The listing builds one solid part. Answer for the finished solid, in the listing's coordinates (mm). A direction names the side the tool comes from. Coordinates: 2 decimals unless noted, no trailing zeros. Order: outer loops, then holes, each group sorted by start corner. A loop starts at its lowest first (then second) coordinate and runs counter-clockwise, first axis right, second up. Notation, with made-up numbers: (70, 59.5) - (111, 59.5) arc R32 cw to (111, 96.5) - close; hole circle Ø2 at (67, 84.25). An arc over 180 degrees is marked (long way). Use a Markdown table: item, result. Add a question column.
Item 1: The part is cut by section B-B, the plane z = 5. Give the vertices of the cut face in (x, y), then the cut area to 3 significant figures.
Item 2: The part is cut by section A-A, the plane x = -33. Give the vertices of the cut face in (y, z), then the cut area to 3 significant figures.
Item 3: Find the intervals of material crossed by line 1 along X through (y, z) = (2.5, 3); line 2 along Y through (x, z) = (37.5, -2.5); line 3 along Y through (x, z) = (18.5, -9), in increasing order.
Item 4: Flat-ended cylindrical pins translate along their axes: P1, Ø3, axis at x = 15.5, z = 22, coming from the +Y side; P2, Ø10, axis at x = -1, y = 31.5, coming from the -Z side; P3, Ø12, axis at x = -4.5, y = 9.5, coming from the +Z side. Find the tip coordinate at first contact, or state that the pin passes through.
Item 5: For faces 1 (the flat face through (-1.29, 7.19, 0.91)), 2 (the flat face through (-10.32, -0.54, 6.53)), 3 (the cylindrical face through (32.9, 3.5, -23.5)), determine the directions among +Z, -Z, +X, -X, +Y, -Y from which every point of the face is accessible in a straight line to the end or side of a thin tool.
Item 6: The part is cut by section D-D, the plane z = 25. Give the vertices of the cut face in (x, y), then the cut area to 3 significant figures.
Item 7: The part is cut by section C-C, the plane y = 3.5. Give the vertices of the cut face in (x, z).
Item 8: The mould has two halves that part along Y. Classify faces 4 (the flat face through (7.42, 17.14, -4.5)), 5 (the flat face through (39, 3, 26)), 6 (the flat face through (-4.37, 22.4, 1.41)), 7 (the flat face through (9.5, 29.32, -7.2)): released by +Y, released by -Y, zero draft, split by the parting line, or undercut.
from build123d import *

# Parameters (mm, degrees)
BOSS_EXTRUDE1_DEPTH = 7
EXTRUDE_THIN1_DEPTH = 7
SKETCH4_R           = 4
BOSS_EXTRUDE2_DEPTH = 4


with BuildPart() as part:
    # Sketch1 → Boss-Extrude1 (new body)
    with BuildSketch(Plane(origin=(0, 0, 0), x_dir=(1, 0, 0), z_dir=(0, 1, 0))):
        Polygon((34, 31), (44, 21), (44, -21), (34, -31), (-34, -31), (-44, -21), (-44, 21), (-34, 31), align=None)
        with BuildLine():
            Line((-30, 20.5), (-30, -20.5))
            ThreePointArc((-30, -20.5), (-33, -23.5), (-36, -20.5))
            Line((-36, -20.5), (-36, 20.5))
            ThreePointArc((-36, 20.5), (-33, 23.5), (-30, 20.5))
        make_face(mode=Mode.SUBTRACT)
        with BuildLine():
            Line((36, 20.5), (36, -20.5))
            ThreePointArc((36, -20.5), (33, -23.5), (30, -20.5))
            Line((30, -20.5), (30, 20.5))
            ThreePointArc((30, 20.5), (33, 23.5), (36, 20.5))
        make_face(mode=Mode.SUBTRACT)
    extrude(amount=BOSS_EXTRUDE1_DEPTH)

    # Sketch3 → Extrude-Thin1 (add, symmetric)
    with BuildSketch(Plane(origin=(0, 0, 0), x_dir=(0.849441251, 0, -0.527683201), z_dir=(0.527683201, 0, 0.849441251))):
        Polygon((-18.849066913, 7), (8.678571497, 27), (8.678571497, 7), (-1.321428503, 7), (-1.321428503, 7.373894945), (-12.97121439, -1.090169944), align=None)
    extrude(amount=EXTRUDE_THIN1_DEPTH, both=True)

    # Sketch4 → Boss-Extrude2 (add)
    with BuildSketch(Plane(origin=(-8.359258135, 13.544823437, 5.192872478), x_dir=(0.866435488, 0.466201263, 0.178734239), z_dir=(-0.49928904, 0.809016994, 0.310164404))):
        with BuildLine():
            Line((20.238219538, 24.365708041), (-17.853578159, -4.883475366))
            Line((-17.853578159, -4.883475366), (-9.327190536, -15.987560835))
            Line((-9.327190536, -15.987560835), (28.764607161, 13.261622572))
            ThreePointArc((28.764607161, 13.261622572), (30.053456084, 23.076859118), (20.238219538, 24.365708041))
        make_face()
        with Locations((24.501413349, 18.813665306)):
            Circle(SKETCH4_R, mode=Mode.SUBTRACT)
    extrude(amount=BOSS_EXTRUDE2_DEPTH)


solid = part.part
Solution:
| question | item | result |
|---|---|---|
| 1 | outline | (-44, 0) - (-36, 0) - (-36, 7) - (-44, 7) - close; (-30, 0) - (-13.1, 0) - (-12.16, -1.09) - (-10.4, 0) - (30, 0) - (30, 7) - (5.22, 7) - (5.22, 26.94) - (-21.31, 10.57) - (-21.31, 7) - (-30, 7) - close; (36, 0) - (44, 0) - (44, 7) - (36, 7) - close; hole (0.94, 7) - (1.55, 7) - (1.55, 7.37) - close |
| 1 | area | 845 mm2 |
| 2 | outline | (0, -31) - (7, -31) - (7, -23.5) - (0, -23.5) - close; (0, 23.5) - (7, 23.5) - (7, 31) - (0, 31) - close |
| 2 | area | 105 mm2 |
| 3 | line 1 | x = -44 to -36, -30 to 30, 36 to 44 |
| 3 | line 2 | y = 0 to 7 |
| 3 | line 3 | y = 0 to 7, 35.56 to 35.74 |
| 4 | P1 | stops at y = 7 |
| 4 | P2 | stops at z = -10.73 |
| 4 | P3 | stops at z = 31 |
| 5 | face 1 | none |
| 5 | face 2 | -Z, +X, -Y |
| 5 | face 3 | +Y, -Y |
| 6 | outline | (-40, 0) - (40, 0) - (40, 7) - (-40, 7) - close |
| 6 | area | 560 mm2 |
| 7 | outline | (-44, -21) - (-34, -31) - (34, -31) - (44, -21) - (44, 21) - (34, 31) - (-34, 31) - (-44, 21) - close; hole (-36, -20.5) arc R3 ccw to (-30, -20.5) - (-30, 20.5) arc R3 ccw to (-36, 20.5) - close; hole (30, -20.5) arc R3 ccw to (36, -20.5) - (36, 20.5) arc R3 ccw to (30, 20.5) - close |
| 8 | face 4 | undercut |
| 8 | face 5 | zero draft |
| 8 | face 6 | released by +Y |
| 8 | face 7 | undercut |
